Part model, mm, in its own coordinate system. Face numbers are marked on the shaded views. A direction names the side the tool comes from. Round coordinates to 2 decimals unless told otherwise and drop trailing zeros. Order: outer loops, then holes, each group sorted by start corner. A loop starts at its lowest first (then second) coordinate and runs counter-clockwise, first axis right, second up. Notation, with made-up numbers: (74, 56.25) -> (99, 56.25) arc R21 ccw to (99, 81.25) -> close; hole circle Ø5 at (-31.5, -38.75). An arc over 180 degrees is marked (long way). Use CSV: the item, a comma, the result in double quotes.
```python
from build123d import *
from OCP.BRepFilletAPI import BRepFilletAPI_MakeChamfer

# Parameters (mm, degrees)
SFAZOWANIE1_SIZE  = 1
SFAZOWANIE1_SIZE2 = 1.017920191


with BuildPart() as part:
    # Szkic1 → Obrót1 (revolve)
    with BuildSketch(Plane.XY, mode=Mode.PRIVATE) as obr_t1_sk:
        with BuildLine():
            Line((-24.45, 14.960440746), (-24.45, 104.960440746))
            Line((-24.45, 104.960440746), (-48, 104.960440746))
            Line((-48, 104.960440746), (-49.832781817, -0.039559254))
            Line((-49.832781817, -0.039559254), (-49.832781817, -6.039559254))
            Line((-49.832781817, -6.039559254), (-23.45, -6.039559254))
            Line((-23.45, -6.039559254), (-23.45, 13.960440746))
            ThreePointArc((-23.45, 13.960440746), (-24.157106781, 14.253333965), (-24.45, 14.960440746))
        make_face()
    revolve(obr_t1_sk.sketch.rotate(Axis((0, 0, 0), (0, 1, 0)), 180), axis=Axis((0, 0, 0), (0, 1, 0)))

    # Sfazowanie1: one chamfer whose edges measure the first distance from different faces: ONE call of the kernel's chamfer builder (chamfer() names one face for all edges)
    sfazowanie1_edges_1 = [part.edges().sort_by_distance(p)[0] for p in [
        (-24.45, 104.960440746, 0),
        (-23.45, -6.039559254, 0),
        (-49.832781817, -6.039559254, 0),
    ]]
    sfazowanie1_edges_2 = [part.edges().sort_by_distance(p)[0] for p in [
        (-48, 104.960440746, 0),
    ]]
    sfazowanie1_side_2 = [part.faces().sort_by_distance(p)[0] for p in [
        (-25.80764502, 104.960440746, 0),
    ]]
    sfazowanie1 = BRepFilletAPI_MakeChamfer(part.part.solid().wrapped)
    for e in sfazowanie1_edges_1:
        sfazowanie1.Add(SFAZOWANIE1_SIZE, e.wrapped)
    for e in sfazowanie1_edges_2:
        sfazowanie1.Add(SFAZOWANIE1_SIZE, SFAZOWANIE1_SIZE2, e.wrapped, sfazowanie1_side_2[0].wrapped)  # the first distance lies on this face
    add(Compound.cast(sfazowanie1.Shape()), mode=Mode.REPLACE)


solid = part.part
```
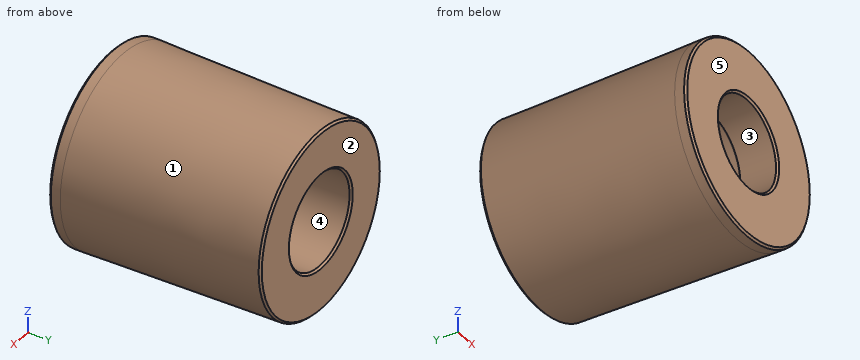
(1) Probe probe 1 along Z at (x, y) = (0, 1.5); probe 2 along X at (y, z) = (51, -7.5); probe 3 along Z at (x, y) = (0, 6.75). List the from-to ranges inside material, lowest first. Write a range as [from, to].
Reply:
probe 1,"[-49.81, -23.45], [23.45, 49.81]"
probe 2,"[-48.36, -23.27], [23.27, 48.36]"
probe 3,"[-49.71, -23.45], [23.45, 49.71]"
(2) Cut at B-B, the plane y = 55. Give the cut face in (x, z), then the cut area to 3 significant figures.
Reply:
outline,"circle Ø97.74 at (0, 0); hole circle Ø48.9 at (0, 0)"
area,"5,630 mm2"
(3) Cut at A-A, the plane y = 25. Give the cut face in (x, z).
Reply:
outline,"circle Ø98.79 at (0, 0); hole circle Ø48.9 at (0, 0)"
(4) Which spindle directions (+Z, -Z, +X, -X, +Y, -Y) get a long thin tool onto all of the face, cutting with end or side? Do the marked faces 4 and 5. Say none if no direction does.
Reply:
face 4,"+Y"
face 5,"+Z, -Z, +X, -X, -Y"
(5) Drop flat-ended pins along their axis: P1, Ø1.5, axis at x = -6.5, y = 17.5, coming from the -Z side; P2, Ø2, axis at y = 30.5, z = 28.5, coming from the +X side; P3, Ø5, axis at x = 0.5, y = 53, coming from the +Z side. Give the stop position or say it passes through.
Reply:
P1,"z = -49.19"
P2,"x = 40.92"
P3,"z = 48.95"
(6) Pull direction Z, two halves, no side cores. Call the marked faces 1, 2 and 3: released by +Z, released by -Z, zero draft, split by the parting line, or undercut.
Reply:
face 1,"split by the parting line"
face 2,"zero draft"
face 3,"undercut"
